from build123d import *

# Parameters (mm, degrees)
SKETCH_1_W          = 25
SKETCH_1_H          = 18
EXTRUDE_1_DEPTH     = 20
CUT_EXTRUDE_1_DEPTH = 20
SKETCH_3_R          = 3
CUT_EXTRUDE_2_DEPTH = 26
CUT_EXTRUDE_3_DEPTH = 21.0000001
SKETCH_5_W          = 23.5
SKETCH_5_H          = 15
CUT_EXTRUDE_4_DEPTH = 18.5
FILLET_1_R          = 1
FILLET_2_R          = 2


with BuildPart() as part:
    # 스케치1 → 보스-돌출1 (new body)
    with BuildSketch(Plane(origin=(0, 0, 0), x_dir=(1, 0, 0), z_dir=(0, 1, 0))):
        with Locations((12.5, 9)):
            Rectangle(SKETCH_1_W, SKETCH_1_H)
    extrude(amount=EXTRUDE_1_DEPTH)

    # 스케치2 → 컷-돌출1 (cut)
    with BuildSketch(Plane.XY):
        with BuildLine():
            ThreePointArc((3, 20), (12.2395604, 9.221784047), (25, 3))
            Line((25, 3), (25, 20))
            Line((25, 20), (3, 20))
        make_face()
        with BuildLine():
            Line((25, 20), (25, 3))
            ThreePointArc((25, 3), (55.118027728, 9.281565928), (68.640222938, 36.916759096))
            ThreePointArc((68.640222938, 36.916759096), (24.905459141, 70.809293693), (3, 20))
            Line((3, 20), (25, 20))
        make_face()
    extrude(amount=-CUT_EXTRUDE_1_DEPTH, mode=Mode.SUBTRACT)

    # 스케치3 → 컷-돌출2 (cut, through all)
    with BuildSketch(Plane.ZY):
        with Locations((-9, 10)):
            Circle(SKETCH_3_R)
    extrude(amount=-CUT_EXTRUDE_2_DEPTH, mode=Mode.SUBTRACT)

    # 스케치4 → 컷-돌출3 (cut, through all)
    with BuildSketch(Plane.XZ):
        with BuildLine():
            Line((11, -6), (14, -6))
            ThreePointArc((14, -6), (17, -9), (14, -12))
            Line((14, -12), (11, -12))
            ThreePointArc((11, -12), (8, -9), (11, -6))
        make_face()
    extrude(amount=-CUT_EXTRUDE_3_DEPTH, mode=Mode.SUBTRACT)

    # 스케치5 → 컷-돌출4 (cut)
    with BuildSketch(Plane(origin=(0, 20, 0), x_dir=(1, 0, 0), z_dir=(0, 1, 0))):
        with Locations((13.25, 9)):
            Rectangle(SKETCH_5_W, SKETCH_5_H)
    extrude(amount=-CUT_EXTRUDE_4_DEPTH, mode=Mode.SUBTRACT)

    # 필렛1
    fillet_1_edges = [part.edges().sort_by_distance(p)[0] for p in [
        (25, 1.5, -9),
        (1.5, 20, -9),
        (1.5, 1.5, -9),
    ]]
    fillet(fillet_1_edges, radius=FILLET_1_R)

    # 필렛2
    fillet_2_edges = [part.edges().sort_by_distance(p)[0] for p in [
        (3, 20, -0.75),
        (25, 3, -17.25),
        (0, 0, -9),
        (3, 20, -17.25),
        (25, 3, -0.75),
    ]]
    fillet(fillet_2_edges, radius=FILLET_2_R)


solid = part.part
Design review of the part built by this model. Coordinates are the model's own, in mm. A direction names the side the tool comes from. Coordinates: 2 decimals unless noted, no trailing zeros. Order: outer loops, then holes, each group sorted by start corner. A loop starts at its lowest first (then second) coordinate and runs counter-clockwise, first axis right, second up. Notation, with made-up numbers: M 50,83 L 83,83 A19 cw 83,93 Z; hole C 55.25,-3.75 d8. An arc over 180 degrees is marked long. Use a Markdown table: item, result.
(1) Wall thickness on probe 1 along Z at (x, y) = (8, 10.5); probe 2 along Y at (x, z) = (20, -2): over which ranges is each line inside the solid? List them lowest first.
Worked answers:
| item | result |
|---|---|
| probe 1 | z = -18 to -16.5, -1.5 to 0 |
| probe 2 | y = 0 to 1.5 |
(2) Add section A-A (x = 9.75). Give the boundary of the cut face in (y, z), then the cut area to 3 significant figures.
Worked answers:
| item | result |
|---|---|
| outline | M 0,-18 L 11.34,-18 L 11.34,-16.5 L 1.5,-16.5 L 1.5,-11.73 L 0,-11.73 Z; M 0,-6.27 L 1.5,-6.27 L 1.5,-1.5 L 11.34,-1.5 L 11.34,0 L 0,0 Z |
| area | 48.3 mm2 |
(3) Add section C-C (z = -10). Give the boundary of the cut face in (x, y), then the cut area to 3 significant figures.
Worked answers:
| item | result |
|---|---|
| outline | M 0,2 A2 ccw 2,0 L 8.17,0 L 8.17,1.5 L 2.5,1.5 A1 cw 1.5,2.5 L 1.5,7.17 L 0,7.17 Z; M 0,12.83 L 1.5,12.83 L 1.5,19 A1 ccw 0.5,20 L 0,20 Z; M 16.83,0 L 25,0 L 25,0.5 A1 ccw 24,1.5 L 16.83,1.5 Z |
| area | 42.7 mm2 |
(4) For faces 1 (the cylindrical face through (8, 1, -9)), 2 (the cylindrical face through (1.785, 1.801, -9.105)), 3 (the cylindrical face through (0.7, 8.2, -11.4)), list the 3-axis set-ups (+Z, -Z, +X, -X, +Y, -Y) from which the entire face can be reached by the end or side of a thin tool; tool diameter is ignored.
Worked answers:
| item | result |
|---|---|
| face 1 | +Y, -Y |
| face 2 | +X, +Y |
| face 3 | +X, -X |
(5) Add section B-B (y = 9). Give the boundary of the cut face in (x, z), then the cut area to 3 significant figures.
Worked answers:
| item | result |
|---|---|
| outline | M 0,-18 L 12.53,-18 L 12.53,-16.5 L 1.5,-16.5 L 1.5,-11.83 L 0,-11.83 Z; M 0,-6.17 L 1.5,-6.17 L 1.5,-1.5 L 12.53,-1.5 L 12.53,0 L 0,0 Z |
| area | 51.6 mm2 |
(6) Draft analysis for pull direction Z (two halves, no side actions). For faces 4 (the flat face through (10, 8, 0)), 5 (the flat face through (0, 13, -11)), 6 (the cylindrical face through (24.715, 1.199, -9.105)), state which applies: released by +Z, released by -Z, zero draft, split by the parting line, or undercut.
Worked answers:
| item | result |
|---|---|
| face 4 | released by +Z |
| face 5 | zero draft |
| face 6 | undercut |
(7) Add section D-D (x = 6.25). Give the boundary of the cut face in (y, z), then the cut area to 3 significant figures.
Worked answers:
| item | result |
|---|---|
| outline | M 0,-18 L 15.13,-18 L 15.13,-16.5 L 1.5,-16.5 L 1.5,-1.5 L 15.13,-1.5 L 15.13,0 L 0,0 Z |
| area | 67.9 mm2 |
(8) For P1, Ø1, axis at x = 20, z = -9.5, coming from the -Y side; P2, Ø3.5, axis at y = 10, z = -9, coming from the -X side; P3, Ø4.5, axis at x = 15, z = -6, coming from the +Y side, all flat-tipped, find the tip position at first contact; note any pin that passes through.
Worked answers:
| item | result |
|---|---|
| P1 | stops at y = 0 |
| P2 | passes through |
| P3 | stops at y = 1.5 |
